from build123d import *

# Parameters (mm, degrees)
BOSS_EXTRUDE1_DEPTH = 10
CUT_EXTRUDE1_START  = 4.5
SKETCH3_R           = 3.05
CUT_EXTRUDE1_DEPTH  = 2


with BuildPart() as part:
    # Sketch1 → Boss-Extrude1 (new body)
    with BuildSketch(Plane.XY):
        with BuildLine():
            Line((-5, 0), (-5, 2))
            add(Edge.make_bspline(
                [(-5, 2), (0, 7), (5, 2)],
                knots=[0, 0, 0, 1, 1, 1], degree=2))
            Line((5, 2), (5, 0))
            add(Edge.make_bspline(
                [(-5, 0), (0, 3), (5, 0)],
                knots=[0, 0, 0, 1, 1, 1], degree=2))
        make_face()
    extrude(amount=BOSS_EXTRUDE1_DEPTH)

    # Sketch3 → Cut-Extrude1 (cut)
    with BuildSketch(Plane(origin=(0, 0, 0), x_dir=(1, 0, 0), z_dir=(0, 1, 0)).offset(CUT_EXTRUDE1_START)):
        with Locations((0, -5)):
            Circle(SKETCH3_R)
    extrude(amount=-CUT_EXTRUDE1_DEPTH, mode=Mode.SUBTRACT)


solid = part.part
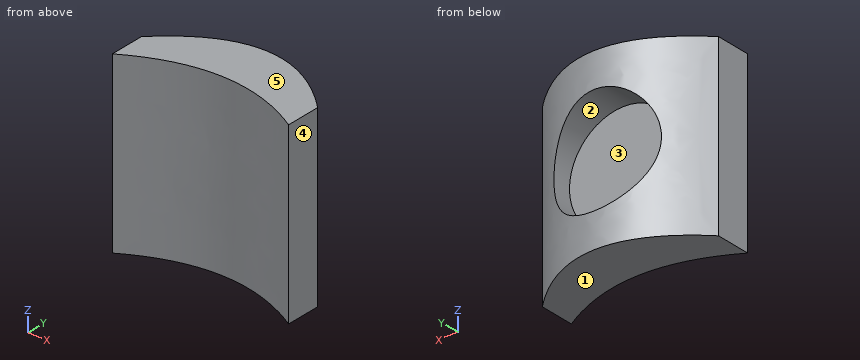
Source: CAD feature listing. Evaluate the final solid. Frame: model axes, mm. Face numbers are marked on the shaded views. A direction names the side the tool comes from. Give positions to 0.01 mm unless a question says otherwise; leave off trailing zeros. Use a Markdown table: item, result. Add a question column.
1) Pull-direction query (X, two-part tool) for the marked faces 3, 4 and 5; classes: +X half, -X half, draft (parallel to the pull), parting line (faces both ways), or undercut.
2) Line query: line 1 along Z through (x, y) = (0, 3.9); line 2 along X through (y, z) = (0.45, 4.5); line 3 along Z through (x, y) = (1, 3.15). Output: solid intervals per line, ascending. Write a range as [from, to].
3) Reachability of the marked faces 1 and 2 from +Z, -Z, +X, -X, +Y, -Y: full face, straight path, thin tool, end or side. Return the list, or none.
4) First-contact query: pin 1 (1.5 mm diameter, centred on x = 1, z = 4, fed in from +Y); pin 2 (4 mm diameter, centred on x = -3, z = 6, fed in from +Y). Flat tips, straight axial feed; report the tip coordinate or a pass-through.
Numbers:
| question | item | result |
|---|---|---|
| 1 | face 3 | undercut |
| 1 | face 4 | +X half |
| 1 | face 5 | draft |
| 2 | line 1 | z = [0, 1.95], [8.05, 10] |
| 2 | line 2 | x = [-5, -4.18], [4.18, 5] |
| 2 | line 3 | z = [0, 2.12], [7.88, 10] |
| 3 | face 1 | -Z, +X, -X, +Y, -Y |
| 3 | face 2 | +Y |
| 4 | pin 1 | stops at y = 2.5 |
| 4 | pin 2 | stops at y = 4.21 |
